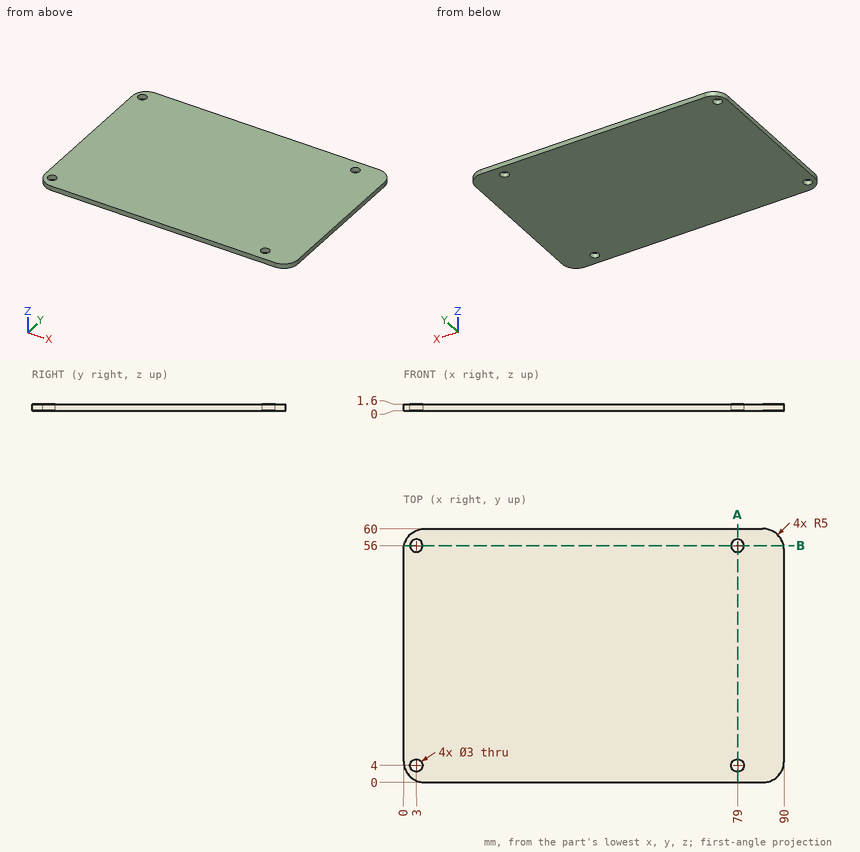
Could you check a few things on this drawing? It's one solid part, dimensions in mm from its lowest x, y, z. Give positions to 0.01 mm unless a question says otherwise; leave off trailing zeros. Write each loop counter-clockwise with the first axis right and the second up, starting at its lowest first coordinate (ties: lowest second). Pieces come first, ordered by that corner, then holes. Notation, with made-up numbers: (-35.75, 88) - (23.25, 88) arc R8 cw to (23.25, 93) - close; hole circle Ø6 at (71, 68.25). An arc over 180 degrees is marked (long way). Use CSV: the item, a comma, the result in double quotes. Start each with the question number.
Item 1: I want a section at A-A, the plane x = 79. Please give me the cut outline in (y, z), then the cut area to 3 significant figures.
Item 2: I want a section at B-B, the plane y = 56. Please give me the cut outline in (x, z).
Item 3: If I drill on line 1 along Y through (x, z) = (79, 0.8), over which ranges is the centre line in solid material (lowest first)?
Item 4: I'm going to push a flat-ended pin straight in: pin 1 (2.5 mm diameter, centred on x = 79, y = 56, fed in from +Z). Where does the tip first touch, or does it pass through?
Findings:
1,outline,"(0, 0) - (2.5, 0) - (2.5, 1.6) - (0, 1.6) - close; (5.5, 0) - (54.5, 0) - (54.5, 1.6) - (5.5, 1.6) - close; (57.5, 0) - (60, 0) - (60, 1.6) - (57.5, 1.6) - close"
1,area,"86.4 mm2"
2,outline,"(0.1, 0) - (1.5, 0) - (1.5, 1.6) - (0.1, 1.6) - close; (4.5, 0) - (77.5, 0) - (77.5, 1.6) - (4.5, 1.6) - close; (80.5, 0) - (89.9, 0) - (89.9, 1.6) - (80.5, 1.6) - close"
3,line 1,"y = 0 to 2.5, 5.5 to 54.5, 57.5 to 60"
4,pin 1,"passes through"
